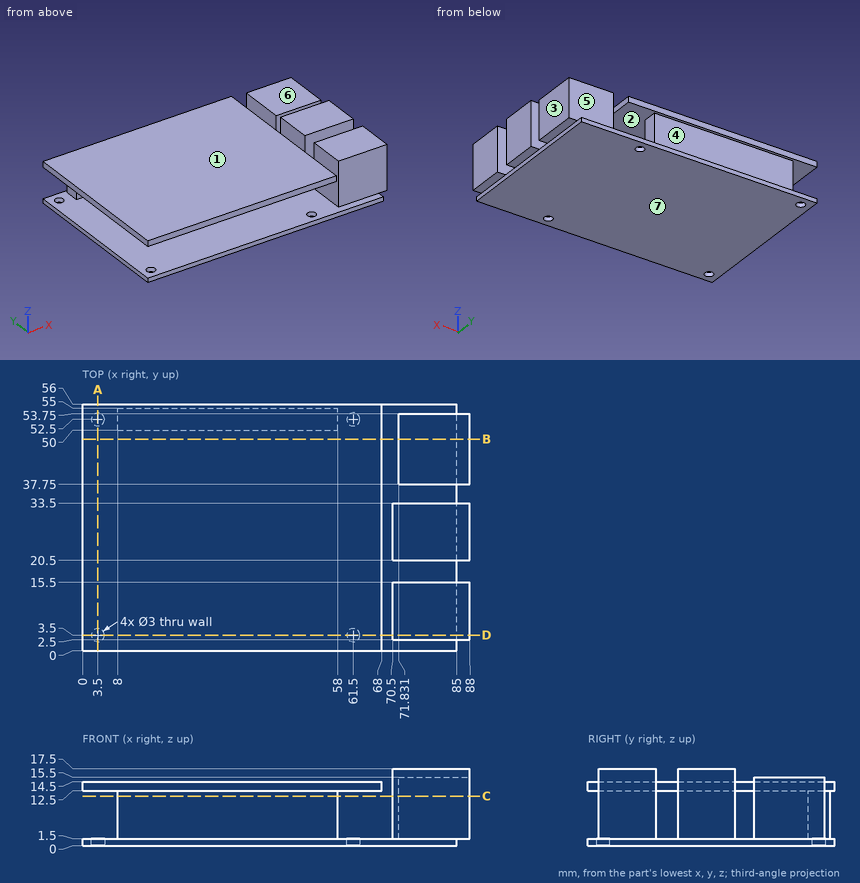
Could you check a few things on this drawing? It's one solid part, dimensions in mm from its lowest x, y, z. A direction names the side the tool comes from. Coordinates: 2 decimals unless noted, no trailing zeros. Loops run counter-clockwise (first coordinate to the right, second up) from the corner with the lowest first, then second, coordinate; pieces in that order, holes last. Notation, with made-up numbers: (-31, -31.75) - (15, -31.75) arc R7 ccw to (15, -25.75) - close; hole circle Ø2 at (38.5, 42.25). An arc over 180 degrees is marked (long way). Return JSON: item names as keys, results as strings. Group by question number.
Item 1: If we section it at B-B on y = 48: Write out the boundary of the cut face in (x, z), and give its area (3 significant figures).
Item 2: Will these pins go through, and if not, where does the flat tip stop? P1, Ø6, axis at x = 38.5, z = 6.5, coming from the -Y side; P2, Ø2.5, axis at x = 61.5, y = 3.5, coming from the +Z side; P3, Ø1, axis at y = 35.5, z = 5, coming from the -X side; P4, Ø1, axis at x = 11, z = 2.5, coming from the +Y side.
Item 3: I need wall thicknesses on line 1 (Y direction, x = 61.5, z = 1.05); line 2 (Z direction, x = 23, y = 39.5); line 3 (Y direction, x = 83, z = 5). Which ranges of each line are inside material? Lowest first, please. Write a range as from..to.
Item 4: If we section it at D-D on y = 3.5: Write out the boundary of the cut face in (x, z).
Item 5: If we section it at C-C on z = 11.25: Write out the boundary of the cut face in (x, y).
Item 6: If we section it at A-A on x = 3.5: Write out the boundary of the cut face in (y, z), and give its area (3 significant figures).
Item 7: We'd pull the mould along Z, two halves only. Please class the marked faces 1, 2, 3 and 4: +Z half, -Z half, draft (parallel to the pull), parting line (faces both ways), or undercut.
Item 8: On a 3-axis mill with a long thin cutter (end or side, diameter ignored), from which of +Z, -Z, +X, -X, +Y, -Y can I reach the whole of each face in a straight line? I mean the marked faces 5, 6 and 7. Say none if no direction works.
Calculated:
{
 "1": {"outline": "(0, 0) - (85, 0) - (85, 1.5) - (88, 1.5) - (88, 15.5) - (71.83, 15.5) - (71.83, 1.5) - (0, 1.5) - close; (0, 12.5) - (68, 12.5) - (68, 14.5) - (0, 14.5) - close", "area": "490 mm^2"},
 "2": {"P1": "stops at y = 50", "P2": "stops at z = 14.5", "P3": "passes through", "P4": "stops at y = 55"},
 "3": {"line 1": "y = 0..2, 5..51, 54..56", "line 2": "z = 0..1.5, 12.5..14.5", "line 3": "y = 2.5..15.5, 20.5..33.5, 37.75..53.75"},
 "4": {"outline": "(0, 0) - (2, 0) - (2, 1.5) - (0, 1.5) - close; (0, 12.5) - (68, 12.5) - (68, 14.5) - (0, 14.5) - close; (5, 0) - (60, 0) - (60, 1.5) - (5, 1.5) - close; (63, 0) - (85, 0) - (85, 1.5) - (88, 1.5) - (88, 17.5) - (70.5, 17.5) - (70.5, 1.5) - (63, 1.5) - close"},
 "5": {"outline": "(8, 50) - (58, 50) - (58, 55) - (8, 55) - close; (70.5, 2.5) - (88, 2.5) - (88, 15.5) - (70.5, 15.5) - close; (70.5, 20.5) - (88, 20.5) - (88, 33.5) - (70.5, 33.5) - close; (71.83, 37.75) - (88, 37.75) - (88, 53.75) - (71.83, 53.75) - close"},
 "6": {"outline": "(0, 0) - (2, 0) - (2, 1.5) - (0, 1.5) - close; (0, 12.5) - (56, 12.5) - (56, 14.5) - (0, 14.5) - close; (5, 0) - (51, 0) - (51, 1.5) - (5, 1.5) - close; (54, 0) - (56, 0) - (56, 1.5) - (54, 1.5) - close", "area": "187 mm^2"},
 "7": {"face 1": "+Z half", "face 2": "undercut", "face 3": "draft", "face 4": "undercut"},
 "8": {"face 5": "+Z, +X, +Y", "face 6": "+Z, +X, -X, +Y", "face 7": "-Z, +X, -X, +Y, -Y"}
}
